Source: CAD feature listing. Evaluate the final solid. Frame: model axes, mm. A direction names the side the tool comes from. Round coordinates to 2 decimals unless told otherwise and drop trailing zeros. Loops run counter-clockwise (first coordinate to the right, second up) from the corner with the lowest first, then second, coordinate; pieces in that order, holes last. Notation, with made-up numbers: M -13,-21.75 L -3,-21.75 A16 cw -3,-1.75 Z; hole C 15,81.25 d6. An arc over 180 degrees is marked long. Answer as a JSON object with one key per item and string values.
from build123d import *

# Parameters (mm, degrees)
SKETCH1_R           = 2.5
SKETCH1_W           = 14
SKETCH1_H           = 14
BOSS_EXTRUDE1_DEPTH = 7


with BuildPart() as part:
    # Sketch1 → Boss-Extrude1 (new body)
    with BuildSketch(Plane(origin=(0, 0, 0), x_dir=(1, 0, 0), z_dir=(0, 1, 0))):
        Polygon((0, 0), (0, 27.5), (-95.593069922, 232.5), (-126, 232.5), (-126, 220), (-140, 220), (-140, 200), (-126, 200), (-126, 187.5), (-106, 187.5), (-43.048466149, 52.5), (-43.048466149, 27.5), (-126, 27.5), (-126, 14), (-140, 14), (-140, 0), align=None)
        with Locations((-102.73, 14)):
            Circle(SKETCH1_R, mode=Mode.SUBTRACT)
        with Locations((-102.73, 210)):
            Circle(SKETCH1_R, mode=Mode.SUBTRACT)
        with Locations((-24.5, 13.75)):
            Rectangle(SKETCH1_W, SKETCH1_H, mode=Mode.SUBTRACT)
    extrude(amount=BOSS_EXTRUDE1_DEPTH)


solid = part.part
Item 1: Contact query for flat-ended pins moving along their axis: pin 1 Ø2 at (x, y) = (-135, 5) entering from -Z; pin 2 Ø3.5 at (y, z) = (2.5, -228.5) entering from -X; pin 3 Ø3 at (y, z) = (3, -123.5) entering from +X; pin 4 Ø3 at (x, z) = (-102.73, -210) entering from -Y. Output: stop coordinate, or through.
Answer sheet:
{"pin 1": "stops at z = -220", "pin 2": "stops at x = -126", "pin 3": "stops at x = -44.07", "pin 4": "passes through"}
Item 2: Pull-direction query (X, two-part tool) for faces 1 (the flat face through (-84, 3, -27.5)), 2 (the flat face through (-25, 3, -6.75)), 3 (the flat face through (0, 3, -14)); classes: pulls with the +X half, pulls with the -X half, needs draft (parallel to the pull), parting line crosses it, or undercut.
Answer sheet:
{"face 1": "needs draft", "face 2": "undercut", "face 3": "pulls with the +X half"}
Item 3: Section C-C on z = -210. Return the cut outline in (x, y).
Answer sheet:
{"outline": "M -140,0 L -105.23,0 L -105.23,7 L -140,7 Z; M -100.23,0 L -85.1,0 L -85.1,7 L -100.23,7 Z"}
Item 4: Line query: probe 1 along Z at (x, y) = (-102.73, 1.5); probe 2 along X at (y, z) = (4.75, -16); probe 3 along Z at (x, y) = (-105, 2). Output: solid intervals per line, ascending. Write a range as from..to.
Answer sheet:
{"probe 1": "z = -232.5..-212.5, -207.5..-180.49, -27.5..-16.5, -11.5..0", "probe 2": "x = -126..-104.23, -101.23..-31.5, -17.5..0", "probe 3": "z = -232.5..-211.05, -208.95..-185.36, -27.5..-15.05, -12.95..0"}
Item 5: Section B-B on y = 3.5. Return the cut outline in (x, z), then the cut area to 3 significant figures.
Answer sheet:
{"outline": "M -140,-220 L -126,-220 L -126,-232.5 L -95.59,-232.5 L 0,-27.5 L 0,0 L -140,0 L -140,-14 L -126,-14 L -126,-27.5 L -43.05,-27.5 L -43.05,-52.5 L -106,-187.5 L -126,-187.5 L -126,-200 L -140,-200 Z; hole C -102.73,-210 d5; hole C -102.73,-14 d5; hole M -31.5,-20.75 L -17.5,-20.75 L -17.5,-6.75 L -31.5,-6.75 Z", "area": "10,700 mm²"}
Item 6: Access query for faces 4 (the flat face through (-71, 3, 0)), 5 (the flat face through (-126, 3, -226)), 6 (the flat face through (-25, 3, -20.75)), 7 (the flat face through (-133, 3, -14)). Directions: +Z, -Z, +X, -X, +Y, -Y. A direction counts if a zero-diameter tool reaches every point of the face in a straight line with its end or side. Return the directions, or none.
Answer sheet:
{"face 4": "+Z, +X, -X, +Y, -Y", "face 5": "-Z, -X, +Y, -Y", "face 6": "+Y, -Y", "face 7": "-X, +Y, -Y"}
Item 7: Section A-A on x = -115. Return the cut outline in (y, z).
Answer sheet:
{"outline": "M 0,-232.5 L 7,-232.5 L 7,-187.5 L 0,-187.5 Z; M 0,-27.5 L 7,-27.5 L 7,0 L 0,0 Z"}
Item 8: Section D-D on z = -36. Return the cut outline in (x, y).
Answer sheet:
{"outline": "M -43.05,0 L -3.96,0 L -3.96,7 L -43.05,7 Z"}
